```python
from build123d import *

# Parameters (mm, degrees)
SKETCH_1_W          = 40
SKETCH_1_H          = 75
EXTRUDE_1_DEPTH     = 21
FILLET_1_R          = 20
CHAMFER_1_SIZE      = 10
EXTRUDE_2_DEPTH     = 700
SKETCH_3_R          = 19
EXTRUDE_4_DEPTH     = 74
SKETCH_4_W          = 17
SKETCH_4_H          = 17
EXTRUDE_5_DEPTH     = 19
SKETCH_5_R          = 3
CUT_EXTRUDE_1_DEPTH = 19
SKETCH_6_R          = 10
EXTRUDE_6_DEPTH     = 16.5
SKETCH_7_R          = 20
EXTRUDE_7_DEPTH     = 20
SKETCH_8_W          = 50
SKETCH_8_H          = 57.5
EXTRUDE_8_DEPTH     = 2
SKETCH_9_W          = 2
SKETCH_9_H          = 57.5
EXTRUDE_9_DEPTH     = 24.5
SKETCH_10_W         = 2
SKETCH_10_H         = 41.5
EXTRUDE_10_DEPTH    = 24.5


with BuildPart() as part:
    # 草图1 → 凸台-拉伸1 (new body)
    with BuildSketch(Plane.XY):
        Rectangle(SKETCH_1_W, SKETCH_1_H)
    extrude(amount=EXTRUDE_1_DEPTH)

    # 圆角1
    fillet_1_edges = [part.edges().sort_by_distance(p)[0] for p in [
        (-20, 37.5, 10.5),
        (20, 37.5, 10.5),
    ]]
    fillet(fillet_1_edges, radius=FILLET_1_R - 0.0001)  # a hair under: the kernel refuses the full size

    # 倒角1
    chamfer_1_edges = [part.edges().sort_by_distance(p)[0] for p in [
        (20, -37.5, 10.5),
        (-20, -37.5, 10.5),
    ]]
    chamfer(chamfer_1_edges, length=CHAMFER_1_SIZE)

    # 草图2 → 凸台-拉伸2 (add)
    with BuildSketch(Plane(origin=(0, 0, 0), x_dir=(-1, 0, 0), z_dir=(0, 0, -1))):
        with BuildLine():
            Line((-10, -37.5), (10, -37.5))
            Line((10, -37.5), (14.449874371, -21.525062814))
            ThreePointArc((14.449874371, -21.525062814), (0, -2.5), (-14.449874371, -21.525062814))
            Line((-14.449874371, -21.525062814), (-10, -37.5))
        make_face()
    extrude(amount=EXTRUDE_2_DEPTH)

    # 草图3 → 凸台-拉伸4 (add)
    with BuildSketch(Plane(origin=(0, 0, 0), x_dir=(-1, 0, 0), z_dir=(0, 0, -1))):
        with Locations(Location((0, 17.5, 0), (0, 0, 180))):
            Circle(SKETCH_3_R)
    extrude(amount=EXTRUDE_4_DEPTH)

    # 草图4 → 凸台-拉伸5 (add)
    with BuildSketch(Plane.XY.offset(21)):
        with Locations((0, -16.5)):
            Rectangle(SKETCH_4_W, SKETCH_4_H)
    extrude(amount=EXTRUDE_5_DEPTH)

    # 草图5 → 切除-拉伸1 (cut)
    with BuildSketch(Plane.ZY.offset(8.5)):
        with Locations(Location((31.5, -16.5, 0), (0, 0, 270))):
            Circle(SKETCH_5_R)
    extrude(amount=-CUT_EXTRUDE_1_DEPTH, mode=Mode.SUBTRACT)

    # 草图6 → 凸台-拉伸6 (add)
    with BuildSketch(Plane(origin=(0, 0, -700), x_dir=(-1, 0, 0), z_dir=(0, 0, -1))):
        with Locations((0, -17.5)):
            Circle(SKETCH_6_R)
    extrude(amount=EXTRUDE_6_DEPTH)

    # 草图7 → 凸台-拉伸7 (add)
    with BuildSketch(Plane(origin=(0, 0, -716.5), x_dir=(-1, 0, 0), z_dir=(0, 0, -1))):
        with Locations((0, -17.5)):
            Circle(SKETCH_7_R)
    extrude(amount=EXTRUDE_7_DEPTH)

    # 草图8 → 凸台-拉伸8 (add)
    with BuildSketch(Plane(origin=(0, 0, -736.5), x_dir=(-1, 0, 0), z_dir=(0, 0, -1))):
        with Locations((0, -17.5)):
            Rectangle(SKETCH_8_W, SKETCH_8_H)
    extrude(amount=EXTRUDE_8_DEPTH)

    # 草图9 → 凸台-拉伸9 (add)
    with BuildSketch(Plane(origin=(0, 0, -738.5), x_dir=(-1, 0, 0), z_dir=(0, 0, -1))):
        with Locations((24, -17.5)):
            Rectangle(SKETCH_9_W, SKETCH_9_H)
    extrude(amount=EXTRUDE_9_DEPTH)

    # 草图10 → 凸台-拉伸10 (add)
    with BuildSketch(Plane(origin=(0, 0, -738.5), x_dir=(-1, 0, 0), z_dir=(0, 0, -1))):
        with Locations((-24, -17.5)):
            Rectangle(SKETCH_10_W, SKETCH_10_H)
    extrude(amount=EXTRUDE_10_DEPTH)


solid = part.part
```
Can you work these out from the model? Positions are in its coordinate system, mm. A direction names the side the tool comes from. Round coordinates to 2 decimals unless told otherwise and drop trailing zeros. Loops run counter-clockwise (first coordinate to the right, second up) from the corner with the lowest first, then second, coordinate; pieces in that order, holes last. Notation, with made-up numbers: M 87.5,-8 L 120.5,-8 A17 ccw 120.5,18 Z; hole C -4,7 d9. An arc over 180 degrees is marked long. Answer as a JSON object with one key per item and string values. Group by question number.
Q1. We'd pull the mould along X, two halves only. Please class faces 1 (the flat face through (-23, -18, -751)), 2 (the flat face through (12.256, -29.401, -345.1)), 3 (the flat face through (0, -25, 30)): +X half, -X half, draft (parallel to the pull), parting line (faces both ways), or undercut.
Q2. Please list where these lines run through material, in increasing order: L1, parallel to Z at x = -2.5, y = 3.5; L2, parallel to Z at x = 2, y = -16; L3, parallel to Y at x = -5, z = 31.
Q3. On a 3-axis mill with a long thin cutter (end or side, diameter ignored), from which of +Z, -Z, +X, -X, +Y, -Y can I reach the whole of each face in a straight line? I mean faces 4 (the flat face through (-4, -8, -716.5)), 5 (the flat face through (23, -18, -751)), 6 (the flat face through (-8.5, -17, 28)). Say none if no direction works.
Q4. Will these pins go through, and if not, where does the flat tip stop? pin 1 (23 mm diameter, centred on y = -15.5, z = 12.5, fed in from -X); pin 2 (4 mm diameter, centred on y = -36, z = -188.5, fed in from -X); pin 3 (7 mm diameter, centred on y = -16.5, z = 31.5, fed in from -X).
Q5. Imagine slicing it at B-B, the plane z = -464.5. Please give me the cut outline in (x, y), then the cut area to 3 significant figures.
Q6. Imagine slicing it at A-A, the plane y = 29.5. Please give me the cut outline in (x, z), then the cut area to 3 significant figures.
Findings:
{
 "1": {"face 1": "undercut", "face 2": "+X half", "face 3": "draft"},
 "2": {"L1": "z = -738.5 to -736.5, -74 to 21", "L2": "z = -738.5 to 28.54, 34.46 to 40", "L3": "y = -25 to -19.46, -13.54 to -8"},
 "3": {"face 4": "none", "face 5": "-Z, +Y, -Y", "face 6": "+Z, -X, +Y, -Y"},
 "4": {"pin 1": "stops at x = -20", "pin 2": "stops at x = -10.97", "pin 3": "stops at x = -8.5"},
 "5": {"outline": "M -14.45,-21.53 L -10,-37.5 L 10,-37.5 L 14.45,-21.53 A15 ccw long Z", "area": "863 mm2"},
 "6": {"outline": "M -16,0 L -14.73,0 L -14.73,-74 L 14.73,-74 L 14.73,0 L 16,0 L 16,21 L -16,21 Z", "area": "2,850 mm2"}
}
